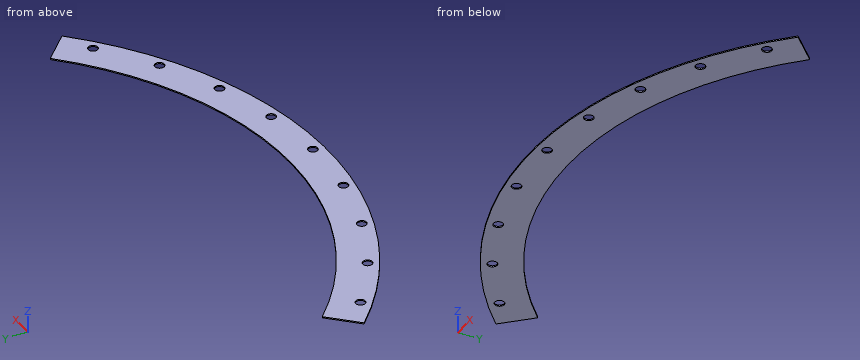
from build123d import *

# Parameters (mm, degrees)
BOSS_EXTRUDE1_DEPTH    = 3.175
F_1_1_DIAMETER_HOLE1_D = 25.4


with BuildPart() as part:
    # Sketch → Boss-Extrude1 (new body)
    with BuildSketch(Plane.XY):
        with BuildLine():
            Line((-647.690106465, -649.9549266), (-719.406658046, -721.922254113))
            ThreePointArc((-719.406658046, -721.922254113), (0, -1019.175), (719.406658046, -721.922254113))
            Line((719.406658046, -721.922254113), (647.690106465, -649.9549266))
            ThreePointArc((647.690106465, -649.9549266), (0, -917.575), (-647.690106465, -649.9549266))
        make_face()
    extrude(amount=BOSS_EXTRUDE1_DEPTH)

    # 1 (1) Diameter Hole1 (through all)
    with Locations(Plane(origin=(-384.964871278, 41.304236103, 3.175), x_dir=(1, 0, 0), z_dir=(0, 0, 1))):
        with Locations((1021.710277433, -800.147861457), (880.264871278, -899.189001092), (723.770025256, -972.163746254), (556.980756074, -1016.854796237), (384.964871278, -1031.904236103), (212.948986481, -1016.854796237), (46.159717299, -972.163746254), (-110.335128722, -899.189001092), (-251.780534878, -800.147861457)):
            Hole(F_1_1_DIAMETER_HOLE1_D / 2)


solid = part.part
Check sheet for the modelled part. Datum: model origin and axes. Units: mm. Round coordinates to 2 decimals unless told otherwise and drop trailing zeros. Loops run counter-clockwise (first coordinate to the right, second up) from the corner with the lowest first, then second, coordinate; pieces in that order, holes last. Notation, with made-up numbers: M 46,26 L 105,26 A32 ccw 105,53 Z; hole C 60.5,-20.75 d1. An arc over 180 degrees is marked long. One line per item, written item: value.
(1) Thickness scan on line 1 (Y direction, x = 628, z = 0.3); line 2 (Y direction, x = -14.5, z = 2.8); line 3 (Y direction, x = 495.3, z = 1.9). Record the ranges inside material, lowest first.
Computed values:
line 1: y = -802.7 to -768.05, -749.63 to -669
line 2: y = -1019.07 to -917.46
line 3: y = -890.73 to -870.58, -845.18 to -772.41
(2) Sectioned sample at C-C, the plane z = 2. Count the separate pieces of the cut face and the enclosed holes in it, then the cut area to 3 significant figures.
Computed values:
separate pieces: 1
enclosed holes: 9
area: 150,000 mm^2
(3) Sectioned sample at D-D, the plane x = 232.5. Record the cut outline in (y, z) (3 decimals), then the cut area to 3 significant figures.
Computed values:
outline: M -992.301,0 L -887.63,0 L -887.63,3.175 L -992.301,3.175 Z
area: 332 mm^2
(4) Sectioned sample at A-A, the plane x = 0. Record the cut outline in (y, z) (3 decimals).
Computed values:
outline: M -1019.175,0 L -1003.3,0 L -1003.3,3.175 L -1019.175,3.175 Z; M -977.9,0 L -917.575,0 L -917.575,3.175 L -977.9,3.175 Z
(5) Sectioned sample at B-B, the plane y = -833. Record the cut outline in (x, z) (3 decimals).
Computed values:
outline: M -587.221,0 L -384.779,0 L -384.779,3.175 L -587.221,3.175 Z; M 384.779,0 L 587.221,0 L 587.221,3.175 L 384.779,3.175 Z
